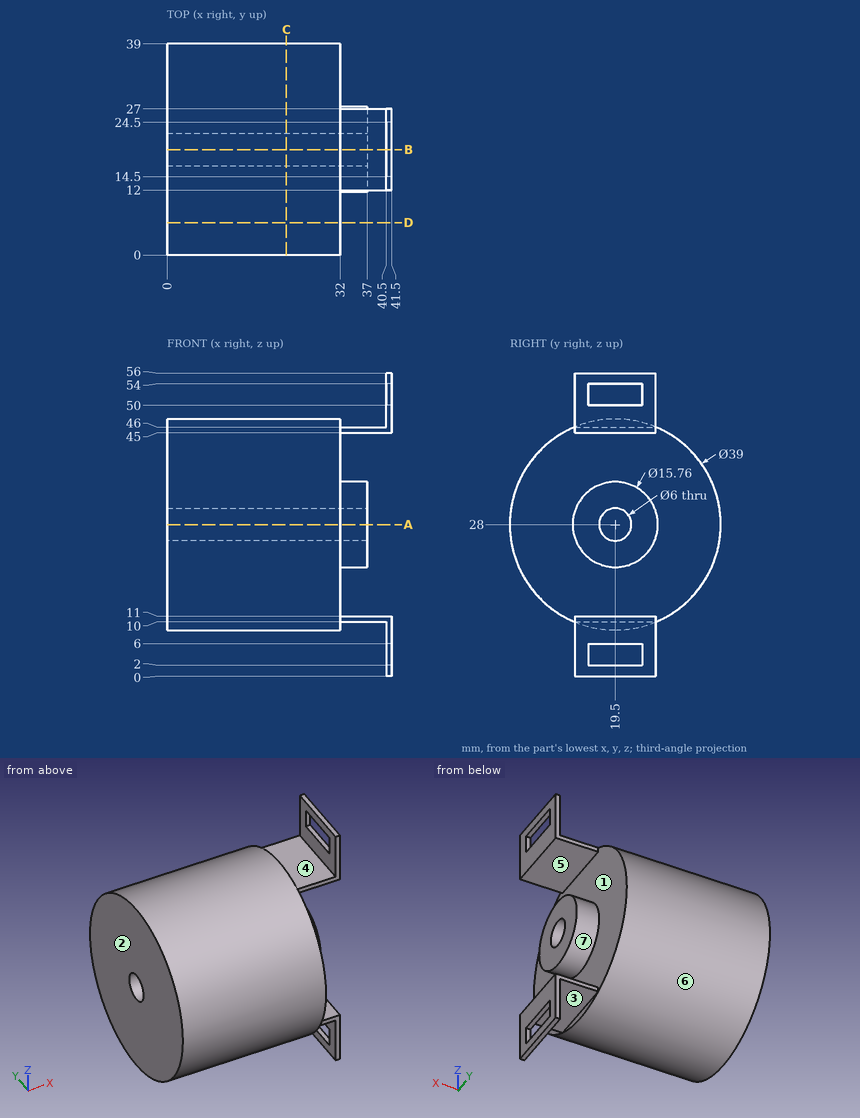
Check sheet for the drawn part. Datum: minimum x, y, z corner. Units: mm. A direction names the side the tool comes from. Coordinates: 2 decimals unless noted, no trailing zeros. Order: outer loops, then holes, each group sorted by start corner. A loop starts at its lowest first (then second) coordinate and runs counter-clockwise, first axis right, second up. Notation, with made-up numbers: M 14.5,-26.75 L 33.5,-26.75 A18 ccw 33.5,6.25 Z; hole C -4.75,41 d4. An arc over 180 degrees is marked long. One line per item, written item: value. Start each with the question number.
Item 1: Sectioned sample at C-C (x = 22). Enter the section's corners in (y, z), then the cut area to 3 significant figures.
Item 2: Sectioned sample at B-B (y = 19.5). Count the separate pieces of the cut face and the enclosed holes in it, then the cut area to 3 significant figures.
Item 3: Sectioned sample at D-D (y = 6). Enter the section's corners in (x, z).
Item 4: Mould release check, pull along Z, two halves, no side actions. Record for the marked faces 1, 2, 3 and 4: released by +Z, released by -Z, zero draft, split by the parting line, or undercut.
Item 5: Access from +Z, -Z, +X, -X, +Y, -Y to the whole of each face (thin tool, end or side, straight path). Record for the marked faces 5, 6 and 7.
Item 6: Sectioned sample at A-A (z = 28). Enter the section's corners in (x, y), then the cut area to 3 significant figures.
Item 7: Gauge pin test, flat ends, axial feed: pin 1 (8 mm diameter, centred on x = 20.5, z = 39, fed in from +Y); pin 2 (5 mm diameter, centred on y = 18.5, z = 5.5, fed in from -X); pin 3 (3 mm diameter, centred on y = 29, z = 46.5, fed in from +X). Record the tip position at first contact, or that the pin passes through.
Item 8: Scan lines: probe 1 along Y at (x, z) = (12, 28); probe 2 along X at (y, z) = (8.5, 35); probe 3 along X at (y, z) = (21, 33.5). Record each from-to range of solid material in increasing order.
Conclusion:
1. outline: C 19.5,28 d39; hole C 19.5,28 d6
1. area: 1,170 mm^2
2. separate pieces: 4
2. enclosed holes: 0
2. area: 1,140 mm^2
3. outline: M 0,13.93 L 32,13.93 L 32,42.07 L 0,42.07 Z
4. face 1: undercut
4. face 2: zero draft
4. face 3: released by -Z
4. face 4: released by +Z
5. face 5: +X, +Y, -Y
5. face 6: -X
5. face 7: +X
6. outline: M 0,0 L 32,0 L 32,11.62 L 37,11.62 L 37,16.5 L 0,16.5 Z; M 0,22.5 L 37,22.5 L 37,27.38 L 32,27.38 L 32,39 L 0,39 Z
6. area: 1,100 mm^2
7. pin 1: stops at y = 37.7
7. pin 2: stops at x = 40.5
7. pin 3: stops at x = 32
8. probe 1: y = 0 to 16.5, 22.5 to 39
8. probe 2: x = 0 to 32
8. probe 3: x = 0 to 37
